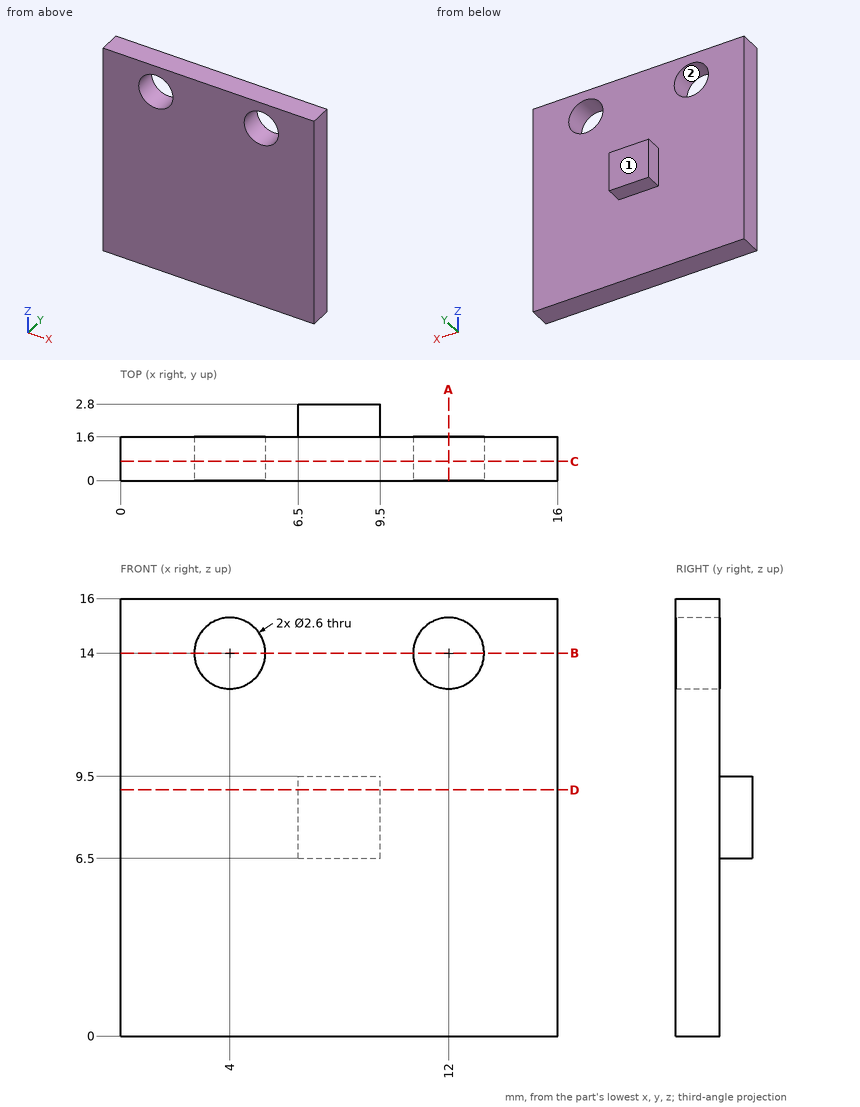
Geometry check sheet. Reference: drawing and pictorial views, mm from the part's lowest x, y, z. Round coordinates to 2 decimals unless told otherwise and drop trailing zeros. Loops run counter-clockwise (first coordinate to the right, second up) from the corner with the lowest first, then second, coordinate; pieces in that order, holes last. Notation, with made-up numbers: (42, -7) -> (55, -7) arc R29 cw to (55, 21) -> close; hole circle Ø4 at (59, 19). An arc over 180 degrees is marked (long way). Answer as a JSON object with one key per item and string values.
Q1. Section check B-B (z = 14). Record the boundary of the cut face in (x, y).
Data:
{"outline": "(0, 0) -> (2.7, 0) -> (2.7, 1.6) -> (0, 1.6) -> close; (5.3, 0) -> (10.7, 0) -> (10.7, 1.6) -> (5.3, 1.6) -> close; (13.3, 0) -> (16, 0) -> (16, 1.6) -> (13.3, 1.6) -> close"}
Q2. Scan lines: line 1 (X direction, y = 0.85, z = 14); line 2 (Z direction, x = 4, y = 0.6); line 3 (Y direction, x = 1.75, z = 6). Record each from-to range of solid material in increasing order. Write a range as from..to.
Data:
{"line 1": "x = 0..2.7, 5.3..10.7, 13.3..16", "line 2": "z = 0..12.7, 15.3..16", "line 3": "y = 0..1.6"}
Q3. Section check A-A (x = 12). Record the boundary of the cut face in (y, z), then the cut area to 3 significant figures.
Data:
{"outline": "(0, 0) -> (1.6, 0) -> (1.6, 12.7) -> (0, 12.7) -> close; (0, 15.3) -> (1.6, 15.3) -> (1.6, 16) -> (0, 16) -> close", "area": "21.4 mm2"}
Q4. Section check C-C (y = 0.7). Record the boundary of the cut face in (x, z).
Data:
{"outline": "(0, 0) -> (16, 0) -> (16, 16) -> (0, 16) -> close; hole circle Ø2.6 at (4, 14); hole circle Ø2.6 at (12, 14)"}
Q5. Section check D-D (z = 9). Record the boundary of the cut face in (x, y), then the cut area to 3 significant figures.
Data:
{"outline": "(0, 0) -> (16, 0) -> (16, 1.6) -> (9.5, 1.6) -> (9.5, 2.8) -> (6.5, 2.8) -> (6.5, 1.6) -> (0, 1.6) -> close", "area": "29.2 mm2"}
Q6. Draft check along Z on the marked faces 1 and 2. Enter one of: pulls with the +Z half, pulls with the -Z half, needs draft (parallel to the pull), parting line crosses it, or undercut.
Data:
{"face 1": "needs draft", "face 2": "undercut"}
Q7. Go/stop test with flat-tipped pins: P1, Ø0.6, axis at x = 7.5, y = 2, coming from the +Z side; P2, Ø0.6, axis at y = 2, z = 8, coming from the -X side. Record where each tip stops, or that it passes through.
Data:
{"P1": "stops at z = 9.5", "P2": "stops at x = 6.5"}
